Read the model definition and answer for the solid it produces. Units are mm, in the model's axes. Coordinates: 2 decimals unless noted, no trailing zeros. Loops run counter-clockwise (first coordinate to the right, second up) from the corner with the lowest first, then second, coordinate; pieces in that order, holes last.
Q1. Section B-B (x = 16.35) is taken. Give the vertices of the cut face in (y, z), then the cut area to 3 significant figures.
Q2. A flat-ended cylindrical pin translates along its axis: P1, Ø10, axis at x = 38, z = -47.5, coming from the -Y side. Find the tip coordinate at first contact, or state that the pin passes through.
Q3. Section A-A (z = -69.5) is taken. Give the vertices of the cut face in (x, y), then the cut area to 3 significant figures.
Q4. Section C-C (y = 0.85) is taken. Count the separate pieces of the cut face and the enclosed holes in it, then the cut area to 3 significant figures.
Q5. Straight lines are drawn through the part: line 1 (X direction, y = 0.75, z = -63); line 2 (X direction, y = 0.2, z = -39). For each, find the intervals that lie inside material, in ascending order.
from build123d import *

# Parameters (mm, degrees)
ESQUISSE1_W        = 86
ESQUISSE1_H        = 76
ESQUISSE1_R        = 1.45
ESQUISSE1_W_2      = 2
ESQUISSE1_H_2      = 4
ESQUISSE1_W_3      = 6.9
ESQUISSE1_H_3      = 6.9
BOSS_EXTRU_1_DEPTH = 3


with BuildPart() as part:
    # Esquisse1 → Boss.-Extru.1 (new body)
    with BuildSketch(Plane(origin=(0, 0, 0), x_dir=(1, 0, 0), z_dir=(0, 1, 0))):
        with Locations((43, 38)):
            Rectangle(ESQUISSE1_W, ESQUISSE1_H)
        with Locations(Location((16.35, 13.25, 0), (0, 0, 270))):
            Circle(ESQUISSE1_R, mode=Mode.SUBTRACT)
        with Locations(Location((78.55, 13.25, 0), (0, 0, 270))):
            Circle(ESQUISSE1_R, mode=Mode.SUBTRACT)
        with Locations(Location((78.55, 62.75, 0), (0, 0, 90))):
            Circle(ESQUISSE1_R, mode=Mode.SUBTRACT)
        with Locations(Location((16.35, 62.75, 0), (0, 0, 90))):
            Circle(ESQUISSE1_R, mode=Mode.SUBTRACT)
        with Locations(Location((3.5, 22.5, 0), (0, 0, 270))):
            Circle(ESQUISSE1_R, mode=Mode.SUBTRACT)
        with Locations(Location((3.5, 53.5, 0), (0, 0, 90))):
            Circle(ESQUISSE1_R, mode=Mode.SUBTRACT)
        with Locations((61.05, 7)):
            Rectangle(ESQUISSE1_W_2, ESQUISSE1_H_2, mode=Mode.SUBTRACT)
        with Locations((16.35, 7)):
            Rectangle(ESQUISSE1_W_2, ESQUISSE1_H_2, mode=Mode.SUBTRACT)
        with Locations((80.55, 38)):
            Rectangle(ESQUISSE1_W_3, ESQUISSE1_H_3, mode=Mode.SUBTRACT)
        with Locations((33.85, 7)):
            Rectangle(ESQUISSE1_W_2, ESQUISSE1_H_2, mode=Mode.SUBTRACT)
        with Locations((5.45, 5.45)):
            Rectangle(ESQUISSE1_W_3, ESQUISSE1_H_3, mode=Mode.SUBTRACT)
        with Locations((33.85, 21)):
            Rectangle(ESQUISSE1_W_2, ESQUISSE1_H_2, mode=Mode.SUBTRACT)
        with Locations((16.35, 21)):
            Rectangle(ESQUISSE1_W_2, ESQUISSE1_H_2, mode=Mode.SUBTRACT)
        with Locations((78.55, 7)):
            Rectangle(ESQUISSE1_W_2, ESQUISSE1_H_2, mode=Mode.SUBTRACT)
        with Locations((78.55, 21)):
            Rectangle(ESQUISSE1_W_2, ESQUISSE1_H_2, mode=Mode.SUBTRACT)
        with Locations((61.05, 21)):
            Rectangle(ESQUISSE1_W_2, ESQUISSE1_H_2, mode=Mode.SUBTRACT)
        with Locations((61.05, 55)):
            Rectangle(ESQUISSE1_W_2, ESQUISSE1_H_2, mode=Mode.SUBTRACT)
        with Locations((78.55, 55)):
            Rectangle(ESQUISSE1_W_2, ESQUISSE1_H_2, mode=Mode.SUBTRACT)
        with Locations((78.55, 69)):
            Rectangle(ESQUISSE1_W_2, ESQUISSE1_H_2, mode=Mode.SUBTRACT)
        with Locations((16.35, 55)):
            Rectangle(ESQUISSE1_W_2, ESQUISSE1_H_2, mode=Mode.SUBTRACT)
        with Locations((33.85, 55)):
            Rectangle(ESQUISSE1_W_2, ESQUISSE1_H_2, mode=Mode.SUBTRACT)
        with Locations((33.85, 69)):
            Rectangle(ESQUISSE1_W_2, ESQUISSE1_H_2, mode=Mode.SUBTRACT)
        with Locations((5.45, 70.55)):
            Rectangle(ESQUISSE1_W_3, ESQUISSE1_H_3, mode=Mode.SUBTRACT)
        with Locations((61.05, 69)):
            Rectangle(ESQUISSE1_W_2, ESQUISSE1_H_2, mode=Mode.SUBTRACT)
        with Locations((16.35, 69)):
            Rectangle(ESQUISSE1_W_2, ESQUISSE1_H_2, mode=Mode.SUBTRACT)
        with Locations((43.55, 55)):
            Rectangle(ESQUISSE1_W_2, ESQUISSE1_H_2, mode=Mode.SUBTRACT)
        with Locations((43.55, 7)):
            Rectangle(ESQUISSE1_W_2, ESQUISSE1_H_2, mode=Mode.SUBTRACT)
        with Locations((43.55, 21)):
            Rectangle(ESQUISSE1_W_2, ESQUISSE1_H_2, mode=Mode.SUBTRACT)
        with Locations((43.55, 69)):
            Rectangle(ESQUISSE1_W_2, ESQUISSE1_H_2, mode=Mode.SUBTRACT)
    extrude(amount=BOSS_EXTRU_1_DEPTH)


solid = part.part
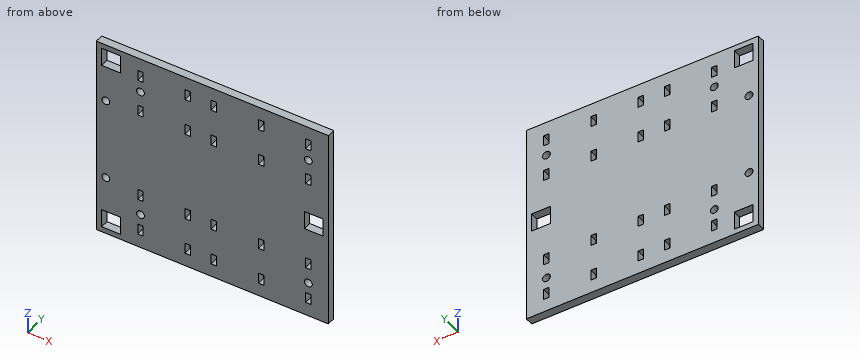
Numbers:
1. outline: (0, -76) - (3, -76) - (3, -71) - (0, -71) - close; (0, -67) - (3, -67) - (3, -64.2) - (0, -64.2) - close; (0, -61.3) - (3, -61.3) - (3, -57) - (0, -57) - close; (0, -53) - (3, -53) - (3, -23) - (0, -23) - close; (0, -19) - (3, -19) - (3, -14.7) - (0, -14.7) - close; (0, -11.8) - (3, -11.8) - (3, -9) - (0, -9) - close; (0, -5) - (3, -5) - (3, 0) - (0, 0) - close
1. area: 163 mm2
2. P1: stops at y = 0
3. outline: (0, 0) - (2, 0) - (2, 3) - (0, 3) - close; (8.9, 0) - (15.35, 0) - (15.35, 3) - (8.9, 3) - close; (17.35, 0) - (32.85, 0) - (32.85, 3) - (17.35, 3) - close; (34.85, 0) - (42.55, 0) - (42.55, 3) - (34.85, 3) - close; (44.55, 0) - (60.05, 0) - (60.05, 3) - (44.55, 3) - close; (62.05, 0) - (77.55, 0) - (77.55, 3) - (62.05, 3) - close; (79.55, 0) - (86, 0) - (86, 3) - (79.55, 3) - close
3. area: 207 mm2
4. separate pieces: 1
4. enclosed holes: 29
4. area: 6,190 mm2
5. line 1: x = 0 to 14.92, 17.78 to 77.12, 79.98 to 86
5. line 2: x = 0 to 77.1, 84 to 86
